Here's the drawing with two shaded views (mm, measured from the low corner). I have some questions. A direction names the side the tool comes from. Give positions to 0.01 mm unless a question says otherwise; leave off trailing zeros. Write each loop counter-clockwise with the first axis right and the second up, starting at its lowest first coordinate (ties: lowest second). Pieces come first, ordered by that corner, then holes.
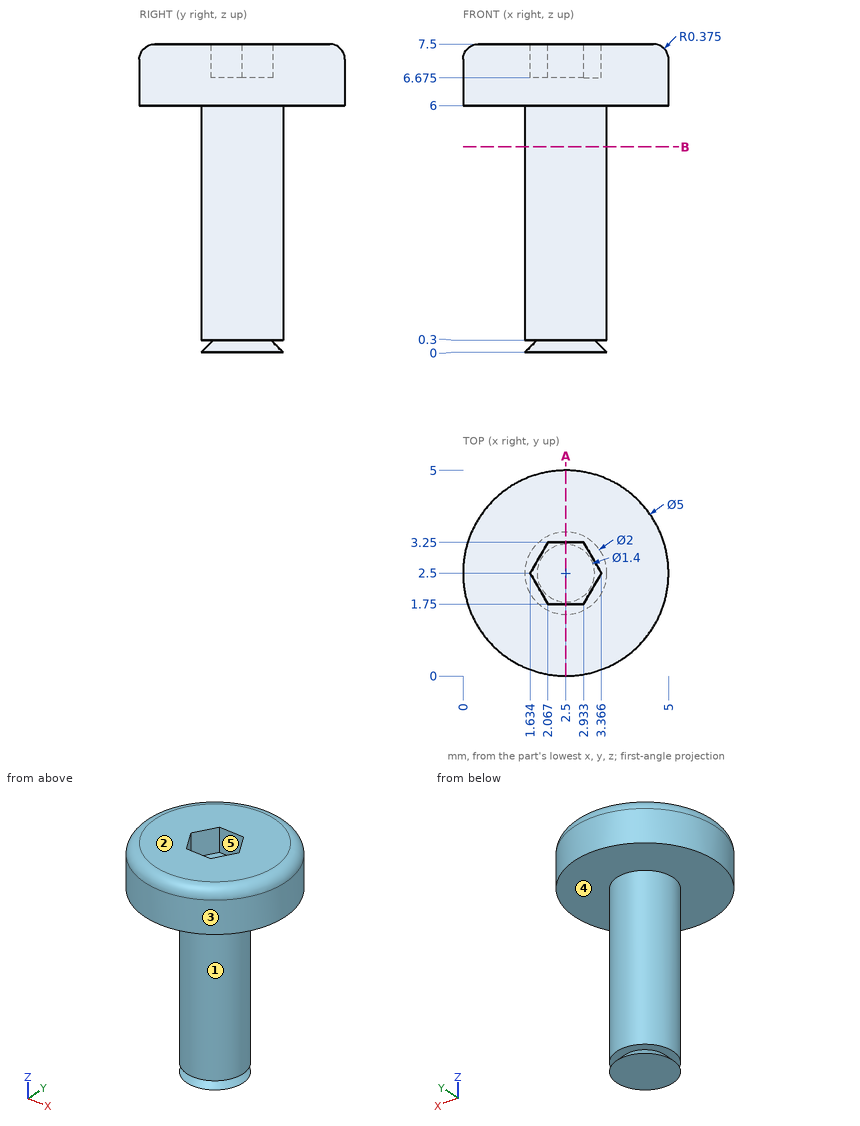
(1) If I drill on L1, parallel to Y at x = 2.5, z = 7; L2, parallel to Z at x = 4.35, y = 1.85; L3, parallel to X at y = 3.4, z = 1.25, over which ranges is the centre line in solid material (lowest first)?
Returned:
L1: y = 0 to 1.75, 3.25 to 5
L2: z = 6 to 7.5
L3: x = 2.06 to 2.94
(2) Imagine slicing it at B-B, the plane z = 5. Write out the boundary of the cut face in (x, y).
Returned:
outline: circle Ø2 at (2.5, 2.5)
(3) If we mould it in two halves opening along X, with no side actions, what happens to the marked faces 3, 4 and 5? For each: +X half, -X half, draft (parallel to the pull), parting line (faces both ways), or undercut.
Returned:
face 3: parting line
face 4: draft
face 5: undercut
(4) For the marked faces 1 and 2, which set-ups out of +Z, -Z, +X, -X, +Y, -Y let a thin tool reach every point of the face, with its end or its side?
Returned:
face 1: -Z
face 2: +Z, +X, -X, +Y, -Y
(5) Will these pins go through, and if not, where does the flat tip stop? P1, Ø2, axis at y = 3.5, z = 3, coming from the +X side; P2, Ø1.5, axis at y = 3.5, z = 6, coming from the -X side.
Returned:
P1: stops at x = 3.5
P2: stops at x = 0.01
(6) Imagine slicing it at A-A, the plane x = 2.5. Write out the boundary of the cut face in (y, z) (3 decimals).
Returned:
outline: (0, 6) - (1.5, 6) - (1.5, 0.3) - (1.8, 0.3) - (1.5, 0) - (3.5, 0) - (3.2, 0.3) - (3.5, 0.3) - (3.5, 6) - (5, 6) - (5, 7.125) arc R0.375 ccw to (4.625, 7.5) - (3.25, 7.5) - (3.25, 6.675) - (1.75, 6.675) - (1.75, 7.5) - (0.375, 7.5) arc R0.375 ccw to (0, 7.125) - close
